Autodesk Inventor part; units mm, degrees
ref_plane "YZ Plane" through (0, 0, 0) normal (1, 0, 0) x (0, 1, 0)
ref_plane "XZ Plane" through (0, 0, 0) normal (0, 1, 0) x (-1, 0, 0)
ref_plane "XY Plane" through (0, 0, 0) normal (0, 0, 1) x (1, 0, 0)
sketch "Sketch1" plane through (0, 0, 0) normal (0, 1, 0) x (-1, 0, 0)
  line L0 (0, 17.4625) -> (0, 1.5875)
  line L1 (1.5875, 0) -> (17.4625, 0)
  line L2 (17.4625, 0) -> (17.4625, -1.5875)
  line L3 (17.4625, -1.5875) -> (-1.5875, -1.5875)
  line L4 (-1.5875, -1.5875) -> (-1.5875, 17.4625)
  line L5 (-1.5875, 17.4625) -> (0, 17.4625)
  arc A0 (0, 1.5875) -> (1.5875, 0) centre (1.5875, 1.5875) ccw
  point P0 (0, 0)
  dimension "d0" = 1.5875
  dimension "d1" = 19.05
  dimension "d2" = 1.5875
extrude "Extrusion1" add sketch "Sketch1" along normal blind 381
sketch "Sketch2" plane through (1.5875, 0, -1.5875) normal (0, 0, -1) x (-1, 0, 0)
  line L0 (19.05, 0) -> (0, 0) construction
  line L1 (9.525, 0) -> (9.525, 443.5725) construction
  circle A0 centre (9.525, 9.525) radius 3.175
  point P0 (1.5875, 0)
  dimension "d5" = 6.35
  dimension "d6" = 9.525
extrude "Extrusion2" cut sketch "Sketch2" against normal through all
sketch "Sketch3" plane through (1.5875, 0, 17.4625) normal (1, 0, 0) x (0, 0, -1)
  line L0 (19.05, 0) -> (0, 0) construction
  line L1 (9.525, 0) -> (9.525, 23.4407) construction
  circle A0 centre (9.525, 9.525) radius 3.175
  point P0 (17.4625, 0)
  dimension "d9" = 6.35
  dimension "d10" = 9.525
extrude "Extrusion3" cut sketch "Sketch3" against normal through all
properties part number "Short Wall support" material "Aluminum 6061"
Build history of the part. All positions in model axes, mm. A direction names the side the tool comes from. Round coordinates to 2 decimals unless told otherwise and drop trailing zeros. Write each loop counter-clockwise with the first axis right and the second up, starting at its lowest first coordinate (ties: lowest second). Pieces come first, ordered by that corner, then holes.
1) Mould opens along Y. For faces 3 (the flat face through (-3.7, 0, -0.5)), 4 (the cylindrical face through (0.805, 12.673, 8.351)), 5 (the flat face through (0, 188, 10)), 6 (the cylindrical face through (-9.644, 12.202, -0.805)) say: +Y half, -Y half, draft (parallel to the pull), parting line (faces both ways), or undercut.
2) Band-saw the part on A-A, the plane y = 207.5. List the corners of the cut face in (x, z) (1 decimal), and give its area (3 significant figures).
3) 3-axis set-ups, long thin cutter, end or side, ignore diameter. For faces 1 (the flat face through (-3.7, 381, -0.5)), 2 (the flat face through (-9, 188, 0)): which of +Z, -Z, +X, -X, +Y, -Y reach the whole face in a straight line?
4) Drill centre lines: probe 1 along X at (y, z) = (161, 3); probe 2 along Z at (x, y) = (-7, 78.5); probe 3 along Z at (x, y) = (-0.25, 200.5). Where is each one in solid material? Low to high.
5) Pin check, flat tips, straight feed: pin 1 (8 mm diameter, centred on x = -8, y = 317.5, fed in from +Z); pin 2 (5 mm diameter, centred on y = 51.5, z = 10.5, fed in from -X). Stop position of each tip, or through.
Ans:
1. face 3: -Y half
1. face 4: undercut
1. face 5: draft
1. face 6: undercut
2. outline: (-17.5, -1.6) - (1.6, -1.6) - (1.6, 17.5) - (0, 17.5) - (0, 1.6) arc R1.6 cw to (-1.6, 0) - (-17.5, 0) - close
2. area: 58.5 mm2
3. face 1: +Z, -Z, +X, -X, +Y
3. face 2: +Z, -X, +Y, -Y
4. probe 1: x = 0 to 1.59
4. probe 2: z = -1.59 to 0
4. probe 3: z = -1.59 to 0.73
5. pin 1: stops at z = 0
5. pin 2: stops at x = 0
